from build123d import *

# Parameters (mm, degrees)
SKETCH1_W           = 222.25
SKETCH1_H           = 88.9
BOSS_EXTRUDE1_DEPTH = 88.9
SKETCH4_W           = 20.32
SKETCH4_H           = 88.9
CUT_EXTRUDE1_DEPTH  = 82.55
SKETCH2_W           = 156.845
SKETCH2_H           = 15.24
SKETCH5_R           = 3.429
CUT_EXTRUDE2_DEPTH  = 183.731111267


with BuildPart() as part:
    # Sketch1 → Boss-Extrude1 (new body)
    with BuildSketch(Plane(origin=(0, 0, 0), x_dir=(1, 0, 0), z_dir=(0, 1, 0))):
        Rectangle(SKETCH1_W, SKETCH1_H)
    extrude(amount=BOSS_EXTRUDE1_DEPTH)

    # Sketch4 → Cut-Extrude1 (cut)
    with BuildSketch(Plane(origin=(0, 88.9, 0), x_dir=(1, 0, 0), z_dir=(0, 1, 0))):
        with Locations((-100.965, 0)):
            Rectangle(SKETCH4_W, SKETCH4_H)
        with Locations((100.965, 0)):
            Rectangle(SKETCH4_W, SKETCH4_H)
    extrude(amount=-CUT_EXTRUDE1_DEPTH, mode=Mode.SUBTRACT)

    # Sketch2 → Revolve1 (revolve)
    with BuildSketch(Plane(origin=(0, 56.1594, 0), x_dir=(1, 0, 0), z_dir=(0, 1, 0))):
        with Locations((-78.4225, 7.62)):
            Rectangle(SKETCH2_W, SKETCH2_H)
    revolve(axis=Axis((0, 56.1594, 0), (-1, 0, 0)))

    # Sketch5 → Cut-Extrude2 (cut, through all)
    with BuildSketch(Plane(origin=(0, 6.35, 0), x_dir=(1, 0, 0), z_dir=(0, 1, 0))):
        with Locations(Location((-98.425, 38.1, 0), (0, 0, 270))):
            Circle(SKETCH5_R)
        with Locations(Location((104.775, 38.1, 0), (0, 0, 270))):
            Circle(SKETCH5_R)
        with Locations(Location((104.775, -38.1, 0), (0, 0, 270))):
            Circle(SKETCH5_R)
        with Locations(Location((-98.425, -38.1, 0), (0, 0, 270))):
            Circle(SKETCH5_R)
    extrude(amount=-CUT_EXTRUDE2_DEPTH, mode=Mode.SUBTRACT)


solid = part.part
Work out the finished part from the listing and answer in its coordinate system (mm). A direction names the side the tool comes from. Round coordinates to 2 decimals unless told otherwise and drop trailing zeros. Write each loop counter-clockwise with the first axis right and the second up, starting at its lowest first coordinate (ties: lowest second). Pieces come first, ordered by that corner, then holes.
1) Straight lines are drawn through the part: line 1 (X direction, y = 2.5, z = 38.1) (3 decimals); line 2 (X direction, y = 4.5, z = 37.5) (3 decimals); line 3 (X direction, y = 79.5, z = 5) (3 decimals). For each, find the intervals that lie inside material, in ascending order.
2) A cutting plane is placed at D-D (y = 20.5). Give the vertices of the cut face in (x, z) (3 decimals), plus the area to 3 significant figures.
3) Given pin 1 Ø5 at (y, z) = (38.5, 33.5) entering from +X (3 decimals); pin 2 Ø6 at (x, z) = (103.5, -12.5) entering from +Y; pin 3 Ø9 at (x, z) = (104.775, -38.1) entering from -Y; pin 4 Ø7 at (y, z) = (2.5, 7.5) entering from -X (3 decimals), each flat-ended and moving along its own axis, determine where each tip first touches the part or whether it passes through.
4) A cutting plane is placed at B-B (x = -108). Give the vertices of the cut face in (y, z).
5) The mould has two halves that part along Z. Classify faces 1 (the cylindrical face through (107.09, 3.22, 35.57)), 2 (the flat face through (-1, 88.9, -1)), 3 (the flat face through (-2, 44, -44.45)): pulls with the +Z half, pulls with the -Z half, needs draft (parallel to the pull), parting line crosses it, or undercut.
6) A cutting plane is placed at A-A (z = -38.1). Give the vertices of the cut face in (x, y) (3 decimals).
7) A cutting plane is placed at C-C (z = 0). Give the vertices of the cut face in (x, y) (3 decimals), plus the area to 3 significant figures.
8) A tool of negligible diameter and unlimited length cuts with its end or side. For faces 4 (the flat face through (-101, 6.35, -1)), 5 (the flat face through (-111.125, 3, 1)), 6 (the flat face through (101, 6.35, -1)), from which of +Z, -Z, +X, -X, +Y, -Y can it reach the whole face along a straight path? Write none if from no direction.
Completed:
1. line 1: x = -111.125 to -101.854, -94.996 to 101.346, 108.204 to 111.125
1. line 2: x = -111.125 to -101.801, -95.049 to 101.399, 108.151 to 111.125
1. line 3: x = -90.805 to 90.805
2. outline: (-90.805, -44.45) - (90.805, -44.45) - (90.805, 44.45) - (-90.805, 44.45) - close
2. area: 16,100 mm2
3. pin 1: stops at x = 90.805
3. pin 2: stops at y = 6.35
3. pin 3: stops at y = 0
3. pin 4: stops at x = -111.125
4. outline: (0, -44.45) - (6.35, -44.45) - (6.35, 44.45) - (0, 44.45) - close; circle Ø30.48 at (56.16, 0)
5. face 1: undercut
5. face 2: needs draft
5. face 3: pulls with the -Z half
6. outline: (-111.125, 0) - (-101.854, 0) - (-101.854, 6.35) - (-111.125, 6.35) - close; (-94.996, 0) - (101.346, 0) - (101.346, 6.35) - (90.805, 6.35) - (90.805, 88.9) - (-90.805, 88.9) - (-90.805, 6.35) - (-94.996, 6.35) - close; (108.204, 0) - (111.125, 0) - (111.125, 6.35) - (108.204, 6.35) - close
7. outline: (-156.845, 40.919) - (-90.805, 40.919) - (-90.805, 6.35) - (-111.125, 6.35) - (-111.125, 0) - (111.125, 0) - (111.125, 6.35) - (90.805, 6.35) - (90.805, 88.9) - (-90.805, 88.9) - (-90.805, 71.399) - (-156.845, 71.399) - close
7. area: 18,400 mm2
8. face 4: +Z, -Z, -X
8. face 5: +Z, -Z, -X, -Y
8. face 6: +Z, -Z, +X, +Y
